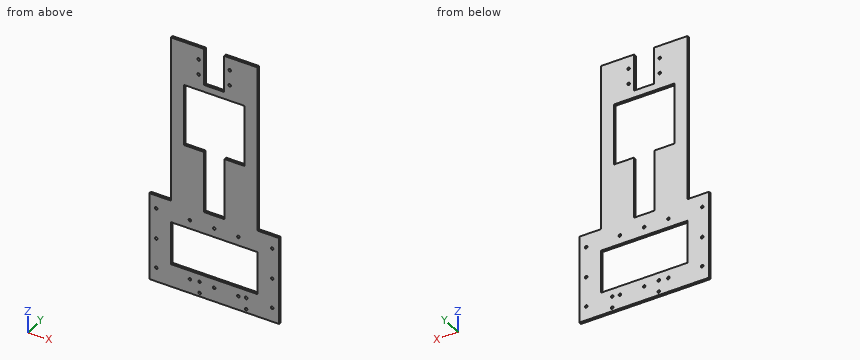
from build123d import *

# Parameters (mm, degrees)
SKETCH_1_R      = 1.5
SKETCH_1_W      = 100
SKETCH_1_H      = 49
EXTRUDE_1_DEPTH = 3


with BuildPart() as part:
    # ｽｹｯﾁ1 → ﾎﾞｽ - 押し出し1 (new body)
    with BuildSketch(Plane.XZ):
        Polygon((61.5, -42), (38.5, -42), (38.5, 0), (0, 0), (0, -190), (-25, -190), (-25, -290), (125, -290), (125, -190), (100, -190), (100, 0), (61.5, 0), align=None)
        with Locations(Location((33.1, -286, 0), (0, 0, 90))):
            Circle(SKETCH_1_R, mode=Mode.SUBTRACT)
        with Locations(Location((86.9, -286, 0), (0, 0, 90))):
            Circle(SKETCH_1_R, mode=Mode.SUBTRACT)
        with Locations(Location((-17, -274, 0), (0, 0, 90))):
            Circle(SKETCH_1_R, mode=Mode.SUBTRACT)
        with Locations(Location((50, -274, 0), (0, 0, 90))):
            Circle(SKETCH_1_R, mode=Mode.SUBTRACT)
        with Locations(Location((117, -274, 0), (0, 0, 90))):
            Circle(SKETCH_1_R, mode=Mode.SUBTRACT)
        with Locations(Location((78, -205, 0), (0, 0, 90))):
            Circle(SKETCH_1_R, mode=Mode.SUBTRACT)
        with Locations(Location((22, -205, 0), (0, 0, 90))):
            Circle(SKETCH_1_R, mode=Mode.SUBTRACT)
        with Locations(Location((68, -14.5, 0), (0, 0, 90))):
            Circle(SKETCH_1_R, mode=Mode.SUBTRACT)
        with Locations(Location((32, -32, 0), (0, 0, 90))):
            Circle(SKETCH_1_R, mode=Mode.SUBTRACT)
        with Locations(Location((32, -14.5, 0), (0, 0, 90))):
            Circle(SKETCH_1_R, mode=Mode.SUBTRACT)
        with Locations(Location((68, -32, 0), (0, 0, 90))):
            Circle(SKETCH_1_R, mode=Mode.SUBTRACT)
        with Locations(Location((-17, -205, 0), (0, 0, 90))):
            Circle(SKETCH_1_R, mode=Mode.SUBTRACT)
        with Locations(Location((50, -205, 0), (0, 0, 90))):
            Circle(SKETCH_1_R, mode=Mode.SUBTRACT)
        with Locations(Location((117, -205, 0), (0, 0, 90))):
            Circle(SKETCH_1_R, mode=Mode.SUBTRACT)
        with Locations(Location((78, -274, 0), (0, 0, 90))):
            Circle(SKETCH_1_R, mode=Mode.SUBTRACT)
        with Locations(Location((22, -274, 0), (0, 0, 90))):
            Circle(SKETCH_1_R, mode=Mode.SUBTRACT)
        with Locations(Location((86.9, -273, 0), (0, 0, 90))):
            Circle(SKETCH_1_R, mode=Mode.SUBTRACT)
        with Locations(Location((33.1, -273, 0), (0, 0, 90))):
            Circle(SKETCH_1_R, mode=Mode.SUBTRACT)
        with Locations(Location((117, -240, 0), (0, 0, 90))):
            Circle(SKETCH_1_R, mode=Mode.SUBTRACT)
        with Locations(Location((-17, -240, 0), (0, 0, 90))):
            Circle(SKETCH_1_R, mode=Mode.SUBTRACT)
        with Locations((50, -239.5)):
            Rectangle(SKETCH_1_W, SKETCH_1_H, mode=Mode.SUBTRACT)
        Polygon((85, -50), (85, -120), (62, -120), (62, -190), (38, -190), (38, -120), (15, -120), (15, -50), align=None, mode=Mode.SUBTRACT)
    extrude(amount=-EXTRUDE_1_DEPTH)


solid = part.part
Input: part model. Units: mm. Frame: model coordinates. Round coordinates to 2 decimals unless told otherwise and drop trailing zeros. Write each loop counter-clockwise with the first axis right and the second up, starting at its lowest first coordinate (ties: lowest second). Pieces come first, ordered by that corner, then holes.
1) Contact query for flat-ended pins moving along their axis: P1, Ø0.9, axis at y = 2, z = -28, coming from the -X side; P2, Ø1.5, axis at x = 70.5, y = 1.5, coming from the +Z side. Output: stop coordinate, or through.
2) Cut plane A-A (z = -84.5). Return the cut outline in (x, y).
3) Ray query, L1, parallel to Z at x = 45, y = 1.85; L2, parallel to Z at x = 86.9, y = 1.4; L3, parallel to Z at x = 68, y = 1.65. Return the intervals inside material, ascending.
4) Cut plane B-B (y = 1.35). Count the separate pieces of the cut face and the enclosed holes in it, then the cut area to 3 significant figures.
Geometry says:
1. P1: stops at x = 0
1. P2: stops at z = 0
2. outline: (0, 0) - (15, 0) - (15, 3) - (0, 3) - close; (85, 0) - (100, 0) - (100, 3) - (85, 3) - close
3. L1: z = -290 to -264, -215 to -190, -50 to -42
3. L2: z = -290 to -287.5, -284.5 to -274.5, -271.5 to -264, -215 to 0
3. L3: z = -290 to -264, -215 to -120, -50 to -33.5, -30.5 to -16, -13 to 0
4. separate pieces: 1
4. enclosed holes: 22
4. area: 21,400 mm2
